Check sheet for the modelled part. Datum: model origin and axes. Units: mm. Face numbers are marked on the shaded views. A direction names the side the tool comes from. Give positions to 0.01 mm unless a question says otherwise; leave off trailing zeros. Order: outer loops, then holes, each group sorted by start corner. A loop starts at its lowest first (then second) coordinate and runs counter-clockwise, first axis right, second up.
```python
from build123d import *

# Parameters (mm, degrees)
F1_DEPTH = 10
F2_R     = 2.25
F3_DEPTH = 5
F4_R     = 2.25
F5_DEPTH = 5


with BuildPart() as f1:
    # F0 (on Top) → F1 (new body, symmetric)
    with BuildSketch(Plane.XY):
        Polygon((4.0990195136, -25), (-0.9009804864, 0), (-40, 0), (-40, -5), (-5, -5), (0, -30), (40, -30), (40, -25), align=None)
    extrude(amount=F1_DEPTH, both=True)

    # F2 (on face) → F3 (cut, through all)
    with BuildSketch(Plane.XZ.offset(5)):
        with Locations((-30, 0)):
            Circle(F2_R)
        with Locations((-10, 0)):
            Circle(F2_R)
    extrude(amount=-F3_DEPTH, mode=Mode.SUBTRACT)

    # F4 (on face) → F5 (cut, through all)
    with BuildSketch(Plane.XZ.offset(30)):
        with Locations((10, 0)):
            Circle(F4_R)
        with Locations((30, 0)):
            Circle(F4_R)
    extrude(amount=-F5_DEPTH, mode=Mode.SUBTRACT)


solid = f1.part
```
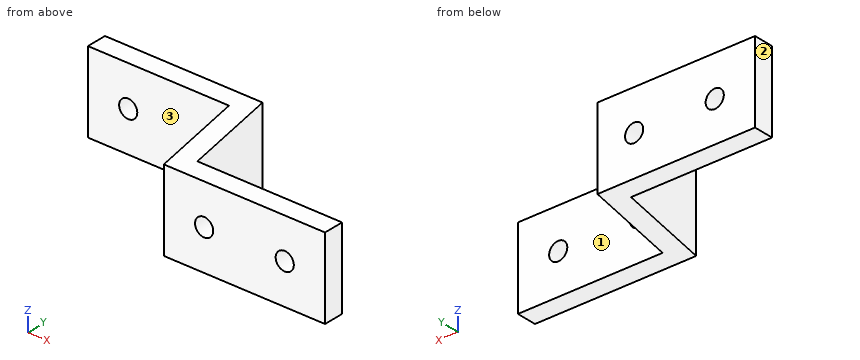
(1) Set-up check for the marked faces 1, 2 and 3: record each of +Z, -Z, +X, -X, +Y, -Y from which the full face is reachable in a straight line by a thin tool's end or side.
Response values:
face 1: +Z, -Z, +X, +Y
face 2: +Z, -Z, -X, +Y, -Y
face 3: +Z, -Z, -X, -Y
(2) Cross-section at C-C on y = -26.75. Enter the section's corners in (x, z), then the cut area to 3 significant figures.
Response values:
outline: (-0.65, -10) - (40, -10) - (40, 10) - (-0.65, 10) - close; hole circle Ø4.5 at (10, 0); hole circle Ø4.5 at (30, 0)
area: 781 mm2
(3) Cross-section at B-B on z = 0. Enter the section's corners in (x, y), then the cut area to 3 significant figures.
Response values:
outline: (-40, -5) - (-32.25, -5) - (-32.25, 0) - (-40, 0) - close; (-27.75, -5) - (-12.25, -5) - (-12.25, 0) - (-27.75, 0) - close; (-7.75, -5) - (-5, -5) - (0, -30) - (7.75, -30) - (7.75, -25) - (4.1, -25) - (-0.9, 0) - (-7.75, 0) - close; (12.25, -30) - (27.75, -30) - (27.75, -25) - (12.25, -25) - close; (32.25, -30) - (40, -30) - (40, -25) - (32.25, -25) - close
area: 412 mm2
(4) Gauge pin test, flat ends, axial feed: pin 1 Ø12 at (y, z) = (-15, -2) entering from +X; pin 2 Ø10 at (x, z) = (-19, 2.5) entering from -Y; pin 3 Ø1.5 at (x, z) = (7, 3) entering from +Y. Record the tip position at first contact, or that the pin passes through.
Response values:
pin 1: stops at x = 3.3
pin 2: stops at y = -5
pin 3: stops at y = -25
(5) Cross-section at A-A on x = -10. Enter the section's corners in (y, z).
Response values:
outline: (-5, -10) - (0, -10) - (0, -2.25) - (-5, -2.25) - close; (-5, 2.25) - (0, 2.25) - (0, 10) - (-5, 10) - close
(6) Material ranges on L1, parallel to Z at x = 10, y = -27.15; L2, parallel to X at y = -2.25, z = 0.5; L3, parallel to Y at x = -35, z = -1, recorded low to high.
Response values:
L1: z = -10 to -2.25, 2.25 to 10
L2: x = -40 to -32.19, -27.81 to -12.19, -7.81 to -0.45
L3: y = -5 to 0
(7) Cross-section at D-D on z = 6.25. Enter the section's corners in (x, y), then the cut area to 3 significant figures.
Response values:
outline: (-40, -5) - (-5, -5) - (0, -30) - (40, -30) - (40, -25) - (4.1, -25) - (-0.9, 0) - (-40, 0) - close
area: 502 mm2
